```python
from build123d import *

# Parameters (mm, degrees)
SKETCH1_W           = 55.88
SKETCH1_H           = 48.26
SKETCH1_R           = 2.65
BOSS_EXTRUDE1_DEPTH = 2.54


with BuildPart() as part:
    # Sketch1 → Boss-Extrude1 (new body)
    with BuildSketch(Plane(origin=(0, 0, 0), x_dir=(1, 0, 0), z_dir=(0, 1, 0))):
        with Locations((22.86, 19.05)):
            Rectangle(SKETCH1_W, SKETCH1_H)
        with Locations(Location((0, 0, 0), (0, 0, 270))):
            Circle(SKETCH1_R, mode=Mode.SUBTRACT)
        with Locations(Location((7.62, 0, 0), (0, 0, 270))):
            Circle(SKETCH1_R, mode=Mode.SUBTRACT)
        with Locations(Location((15.24, 0, 0), (0, 0, 270))):
            Circle(SKETCH1_R, mode=Mode.SUBTRACT)
        with Locations(Location((22.86, 0, 0), (0, 0, 270))):
            Circle(SKETCH1_R, mode=Mode.SUBTRACT)
        with Locations(Location((30.48, 0, 0), (0, 0, 270))):
            Circle(SKETCH1_R, mode=Mode.SUBTRACT)
        with Locations(Location((38.1, 0, 0), (0, 0, 270))):
            Circle(SKETCH1_R, mode=Mode.SUBTRACT)
        with Locations(Location((45.72, 0, 0), (0, 0, 270))):
            Circle(SKETCH1_R, mode=Mode.SUBTRACT)
        with Locations(Location((7.62, 7.62, 0), (0, 0, 270))):
            Circle(SKETCH1_R, mode=Mode.SUBTRACT)
        with Locations(Location((15.24, 7.62, 0), (0, 0, 270))):
            Circle(SKETCH1_R, mode=Mode.SUBTRACT)
        with Locations(Location((22.86, 7.62, 0), (0, 0, 270))):
            Circle(SKETCH1_R, mode=Mode.SUBTRACT)
        with Locations(Location((30.48, 7.62, 0), (0, 0, 270))):
            Circle(SKETCH1_R, mode=Mode.SUBTRACT)
        with Locations(Location((38.1, 7.62, 0), (0, 0, 270))):
            Circle(SKETCH1_R, mode=Mode.SUBTRACT)
        with Locations(Location((45.72, 7.62, 0), (0, 0, 270))):
            Circle(SKETCH1_R, mode=Mode.SUBTRACT)
        with Locations(Location((7.62, 15.24, 0), (0, 0, 270))):
            Circle(SKETCH1_R, mode=Mode.SUBTRACT)
        with Locations(Location((15.24, 15.24, 0), (0, 0, 270))):
            Circle(SKETCH1_R, mode=Mode.SUBTRACT)
        with Locations(Location((22.86, 15.24, 0), (0, 0, 270))):
            Circle(SKETCH1_R, mode=Mode.SUBTRACT)
        with Locations(Location((30.48, 15.24, 0), (0, 0, 270))):
            Circle(SKETCH1_R, mode=Mode.SUBTRACT)
        with Locations(Location((38.1, 15.24, 0), (0, 0, 270))):
            Circle(SKETCH1_R, mode=Mode.SUBTRACT)
        with Locations(Location((45.72, 15.24, 0), (0, 0, 270))):
            Circle(SKETCH1_R, mode=Mode.SUBTRACT)
        with Locations(Location((7.62, 22.86, 0), (0, 0, 270))):
            Circle(SKETCH1_R, mode=Mode.SUBTRACT)
        with Locations(Location((15.24, 22.86, 0), (0, 0, 270))):
            Circle(SKETCH1_R, mode=Mode.SUBTRACT)
        with Locations(Location((22.86, 22.86, 0), (0, 0, 270))):
            Circle(SKETCH1_R, mode=Mode.SUBTRACT)
        with Locations(Location((30.48, 22.86, 0), (0, 0, 270))):
            Circle(SKETCH1_R, mode=Mode.SUBTRACT)
        with Locations(Location((38.1, 22.86, 0), (0, 0, 270))):
            Circle(SKETCH1_R, mode=Mode.SUBTRACT)
        with Locations(Location((45.72, 22.86, 0), (0, 0, 270))):
            Circle(SKETCH1_R, mode=Mode.SUBTRACT)
        with Locations(Location((7.62, 30.48, 0), (0, 0, 270))):
            Circle(SKETCH1_R, mode=Mode.SUBTRACT)
        with Locations(Location((15.24, 30.48, 0), (0, 0, 270))):
            Circle(SKETCH1_R, mode=Mode.SUBTRACT)
        with Locations(Location((22.86, 30.48, 0), (0, 0, 270))):
            Circle(SKETCH1_R, mode=Mode.SUBTRACT)
        with Locations(Location((30.48, 30.48, 0), (0, 0, 270))):
            Circle(SKETCH1_R, mode=Mode.SUBTRACT)
        with Locations(Location((38.1, 30.48, 0), (0, 0, 270))):
            Circle(SKETCH1_R, mode=Mode.SUBTRACT)
        with Locations(Location((45.72, 30.48, 0), (0, 0, 270))):
            Circle(SKETCH1_R, mode=Mode.SUBTRACT)
        with Locations(Location((7.62, 38.1, 0), (0, 0, 270))):
            Circle(SKETCH1_R, mode=Mode.SUBTRACT)
        with Locations(Location((15.24, 38.1, 0), (0, 0, 270))):
            Circle(SKETCH1_R, mode=Mode.SUBTRACT)
        with Locations(Location((22.86, 38.1, 0), (0, 0, 270))):
            Circle(SKETCH1_R, mode=Mode.SUBTRACT)
        with Locations(Location((30.48, 38.1, 0), (0, 0, 270))):
            Circle(SKETCH1_R, mode=Mode.SUBTRACT)
        with Locations(Location((38.1, 38.1, 0), (0, 0, 270))):
            Circle(SKETCH1_R, mode=Mode.SUBTRACT)
        with Locations(Location((45.72, 38.1, 0), (0, 0, 270))):
            Circle(SKETCH1_R, mode=Mode.SUBTRACT)
        with Locations(Location((0, 7.62, 0), (0, 0, 270))):
            Circle(SKETCH1_R, mode=Mode.SUBTRACT)
        with Locations(Location((0, 15.24, 0), (0, 0, 270))):
            Circle(SKETCH1_R, mode=Mode.SUBTRACT)
        with Locations(Location((0, 22.86, 0), (0, 0, 270))):
            Circle(SKETCH1_R, mode=Mode.SUBTRACT)
        with Locations(Location((0, 30.48, 0), (0, 0, 270))):
            Circle(SKETCH1_R, mode=Mode.SUBTRACT)
        with Locations(Location((0, 38.1, 0), (0, 0, 270))):
            Circle(SKETCH1_R, mode=Mode.SUBTRACT)
    extrude(amount=BOSS_EXTRUDE1_DEPTH)


solid = part.part
```
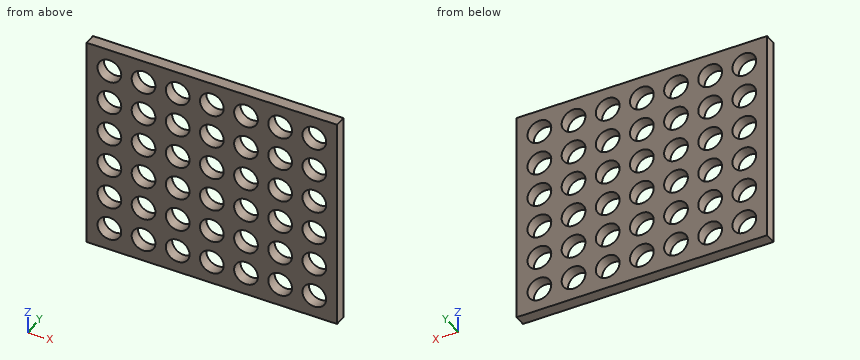
Input: part model. Units: mm. Frame: model coordinates. Give positions to 0.01 mm unless a question says otherwise; leave off trailing zeros. Loops run counter-clockwise (first coordinate to the right, second up) from the corner with the lowest first, then second, coordinate; pieces in that order, holes last. Notation, with made-up numbers: (85, -9) -> (133, -9) arc R31 ccw to (133, 22) -> close; hole circle Ø8 at (-30.75, 53). An arc over 180 degrees is marked (long way). Use a Markdown table: item, result.
Q1. Section query B-B, the plane z = -7.62. State how many separate pieces and enclosed holes the cut face has, plus the area to 3 significant figures.
Entries:
| item | result |
|---|---|
| separate pieces | 8 |
| enclosed holes | 0 |
| area | 47.7 mm² |
Q2. Section query A-A, the plane x = 45.72. Return the cut outline in (y, z).
Entries:
| item | result |
|---|---|
| outline | (0, -43.18) -> (2.54, -43.18) -> (2.54, -40.75) -> (0, -40.75) -> close; (0, -35.45) -> (2.54, -35.45) -> (2.54, -33.13) -> (0, -33.13) -> close; (0, -27.83) -> (2.54, -27.83) -> (2.54, -25.51) -> (0, -25.51) -> close; (0, -20.21) -> (2.54, -20.21) -> (2.54, -17.89) -> (0, -17.89) -> close; (0, -12.59) -> (2.54, -12.59) -> (2.54, -10.27) -> (0, -10.27) -> close; (0, -4.97) -> (2.54, -4.97) -> (2.54, -2.65) -> (0, -2.65) -> close; (0, 2.65) -> (2.54, 2.65) -> (2.54, 5.08) -> (0, 5.08) -> close |
Q3. Section query D-D, the plane x = 14. Return the cut outline in (y, z), plus the area to 3 significant figures.
Entries:
| item | result |
|---|---|
| outline | (0, -43.18) -> (2.54, -43.18) -> (2.54, -40.44) -> (0, -40.44) -> close; (0, -35.76) -> (2.54, -35.76) -> (2.54, -32.82) -> (0, -32.82) -> close; (0, -28.14) -> (2.54, -28.14) -> (2.54, -25.2) -> (0, -25.2) -> close; (0, -20.52) -> (2.54, -20.52) -> (2.54, -17.58) -> (0, -17.58) -> close; (0, -12.9) -> (2.54, -12.9) -> (2.54, -9.96) -> (0, -9.96) -> close; (0, -5.28) -> (2.54, -5.28) -> (2.54, -2.34) -> (0, -2.34) -> close; (0, 2.34) -> (2.54, 2.34) -> (2.54, 5.08) -> (0, 5.08) -> close |
| area | 51.2 mm² |
Q4. First-contact query: P1, Ø8.5, axis at x = 0, z = 0, coming from the -Y side; P2, Ø4, axis at x = 22.86, z = 0, coming from the -Y side. Flat tips, straight axial feed; report the tip coordinate or a pass-through.
Entries:
| item | result |
|---|---|
| P1 | stops at y = 0 |
| P2 | passes through |
